For this review, take the finished solid that the model builds, in its own axes (mm). A direction names the side the tool comes from. Give positions to 0.01 mm unless a question says otherwise; leave off trailing zeros. Loops run counter-clockwise (first coordinate to the right, second up) from the corner with the lowest first, then second, coordinate; pieces in that order, holes last. Notation, with made-up numbers: M 81,86.5 L 105,86.5 A33 ccw 105,119.5 Z; hole C -30,-37.5 d5. An arc over 180 degrees is marked long. Use CSV: the item, a comma, the result in double quotes. Start each with the question number.
1. Take a section at A-A, the plane x = -11.5. Write out the cut boundary in (y, z), and give its area (3 significant figures).
2. The part is to be moulded in two halves that separate along Z. For faces 1 (the face through (-11.43, 1.52, 13.5)), 2 (the face through (-20, 2, 0)), 3 (the face through (-2.6, 19.9, -25)), say which applies: pulls with the +Z half, pulls with the -Z half, needs draft (parallel to the pull), parting line crosses it, or undercut.
3. To check wall thickness, follow line 1 (Y direction, x = -4, z = -17.5); line 2 (X direction, y = 44.5, z = 8); line 3 (X direction, y = 1, z = -15). State the ranges of each line that lie inside material, in increasing order. Write a range as [from, to].
4. Take a section at B-B, the plane z = -15. Write out the cut boundary in (x, y), and give its area (3 significant figures).
5. Insertion check: P1, Ø3, axis at x = -13, z = -9, coming from the +Y side; P2, Ø24, axis at y = 38, z = 2.5, coming from the -X side; P3, Ø2, axis at x = -4, z = 15.5, coming from the -Y side. Each pin has a flat end and moves straight along its axis. Give the tip position at first contact, or say it passes through.
6. Take a section at D-D, the plane x = -16. Write out the cut boundary in (y, z), and give its area (3 significant figures).
7. Tool access review of faces 4 (the face through (0, 27, 0)), 5 (the face through (-11, 3, 0)): name each direction out of +Z, -Z, +X, -X, +Y, -Y from which nothing blocks a thin tool from reaching the whole face with its end or side.
8. Take a section at C-C, the plane z = 0.5. Write out the cut boundary in (x, y).
from build123d import *

# Parameters (mm, degrees)
BOSS_EXTRU_1_DEPTH      = 25
ESQUISSE2_R             = 1.5
ENL_V_MAT_EXTRU_1_DEPTH = 50


with BuildPart() as part:
    # Esquisse1 → Boss.-Extru.1 (new, symmetric)
    with BuildSketch(Plane.XY):
        with BuildLine():
            Line((-20, 0), (-3, 0))
            ThreePointArc((-3, 0), (-0.878679656, 0.878679656), (0, 3))
            Line((0, 3), (0, 50.87))
            Line((0, 50.87), (-3, 50.87))
            Line((-3, 50.87), (-3, 3))
            Line((-3, 3), (-20, 3))
            Line((-20, 3), (-20, 0))
        make_face()
    extrude(amount=BOSS_EXTRU_1_DEPTH, both=True)

    # Esquisse2 → Enlèv. mat.-Extru.1 (cut)
    with BuildSketch(Plane(origin=(0, 3, 0), x_dir=(1, 0, 0), z_dir=(0, 1, 0))):
        with Locations(Location((-11.5, 15, 0), (0, 0, 270))):
            Circle(ESQUISSE2_R)
        with Locations(Location((-11.5, -15, 0), (0, 0, 270))):
            Circle(ESQUISSE2_R)
    extrude(amount=-ENL_V_MAT_EXTRU_1_DEPTH, mode=Mode.SUBTRACT)


solid = part.part
Result set:
1,outline,"M 0,-25 L 3,-25 L 3,-16.5 L 0,-16.5 Z; M 0,-13.5 L 3,-13.5 L 3,13.5 L 0,13.5 Z; M 0,16.5 L 3,16.5 L 3,25 L 0,25 Z"
1,area,"132 mm2"
2,face 1,"undercut"
2,face 2,"needs draft"
2,face 3,"pulls with the -Z half"
3,line 1,"[0, 3]"
3,line 2,"[-3, 0]"
3,line 3,"[-20, -13], [-10, -0.76]"
4,outline,"M -20,0 L -13,0 L -13,3 L -20,3 Z; M -10,0 L -3,0 A3 ccw 0,3 L 0,50.87 L -3,50.87 L -3,3 L -10,3 Z"
4,area,"193 mm2"
5,P1,"y = 3"
5,P2,"x = -3"
5,P3,"y = 0"
6,outline,"M 0,-25 L 3,-25 L 3,25 L 0,25 Z"
6,area,"150 mm2"
7,face 4,"+Z, -Z, +X, +Y, -Y"
7,face 5,"+Z, -Z, -X, +Y"
8,outline,"M -20,0 L -3,0 A3 ccw 0,3 L 0,50.87 L -3,50.87 L -3,3 L -20,3 Z"
